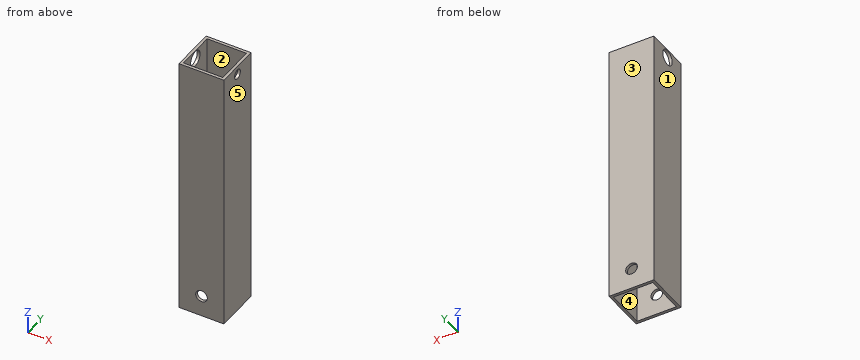
```python
from build123d import *

# Parameters (mm, degrees)
SKETCH1_W                      = 25.4
SKETCH1_H                      = 25.4
BOSS_EXTRUDE1_DEPTH            = 74.93
SHELL1_T                       = -1.5875
CBORE_FOR_M5_SHCS1_D           = 5.5
CBORE_FOR_M5_SHCS1_CBORE_D     = 8.8
CBORE_FOR_M5_SHCS1_CBORE_DEPTH = 5
M6_CLEARANCE_HOLE1_D           = 6.6


with BuildPart() as part:
    # Sketch1 → Boss-Extrude1 (new body, symmetric)
    with BuildSketch(Plane.XY):
        Rectangle(SKETCH1_W, SKETCH1_H)
    extrude(amount=BOSS_EXTRUDE1_DEPTH, both=True)

    # Shell1
    shell1_openings = [part.faces().sort_by_distance(p)[0] for p in [
        (0, 0, 74.93),
        (0, 0, -74.93),
    ]]
    offset(amount=SHELL1_T, openings=shell1_openings, kind=Kind.INTERSECTION)

    # CBORE for M5 SHCS1 (through all)
    with Locations(Plane.ZY.offset(12.7)):
        with Locations((70.1675, 0)):
            CounterBoreHole(CBORE_FOR_M5_SHCS1_D / 2, CBORE_FOR_M5_SHCS1_CBORE_D / 2, CBORE_FOR_M5_SHCS1_CBORE_DEPTH)

    # M6 Clearance Hole1 (through all)
    with Locations(Plane(origin=(0, -12.7, 0), x_dir=(-1, 0, 0), z_dir=(0, -1, 0))):
        with Locations((0, 62.93)):
            Hole(M6_CLEARANCE_HOLE1_D / 2)


solid = part.part
```
Can you work these out from the model? Positions are in its coordinate system, mm. Face numbers are marked on the shaded views. A direction names the side the tool comes from. Coordinates: 2 decimals unless noted, no trailing zeros. Loops run counter-clockwise (first coordinate to the right, second up) from the corner with the lowest first, then second, coordinate; pieces in that order, holes last.
Item 1: If we mould it in two halves opening along X, with no side actions, what happens to the marked faces 3, 4 and 5? For each: released by +X, released by -X, zero draft, split by the parting line, or undercut.
Answers below:
face 3: zero draft
face 4: undercut
face 5: released by +X
Item 2: Please list where these lines run through material, in increasing order: L1, parallel to Y at x = -11, z = -12; L2, parallel to X at y = 11.9, z = -62.93.
Answers below:
L1: y = -12.7 to -11.11, 11.11 to 12.7
L2: x = -12.7 to -3.3, 3.3 to 12.7
Item 3: Suppose I cut it at D-D (z = 64.5). Please give me the cut outline in (x, y), then the cut area to 3 significant figures.
Answers below:
outline: (-12.7, -12.7) - (12.7, -12.7) - (12.7, 12.7) - (-12.7, 12.7) - close; hole (-11.11, -11.11) - (11.11, -11.11) - (11.11, 11.11) - (-11.11, 11.11) - close
area: 151 mm2
Item 4: Suppose I cut it at C-C (y = 0). Please give me the cut outline in (x, z).
Answers below:
outline: (-12.7, -74.93) - (-11.11, -74.93) - (-11.11, 65.77) - (-12.7, 65.77) - close; (-12.7, 74.57) - (-11.11, 74.57) - (-11.11, 74.93) - (-12.7, 74.93) - close; (11.11, -74.93) - (12.7, -74.93) - (12.7, 67.42) - (11.11, 67.42) - close; (11.11, 72.92) - (12.7, 72.92) - (12.7, 74.93) - (11.11, 74.93) - close
Item 5: Suppose I cut it at A-A (x = 0). Please give me the cut outline in (y, z), then the cut area to 3 significant figures.
Answers below:
outline: (-12.7, -74.93) - (-11.11, -74.93) - (-11.11, -66.23) - (-12.7, -66.23) - close; (-12.7, -59.63) - (-11.11, -59.63) - (-11.11, 74.93) - (-12.7, 74.93) - close; (11.11, -74.93) - (12.7, -74.93) - (12.7, -66.23) - (11.11, -66.23) - close; (11.11, -59.63) - (12.7, -59.63) - (12.7, 74.93) - (11.11, 74.93) - close
area: 455 mm2
Item 6: Suppose I cut it at B-B (z = -62.93). Please give me the cut outline in (x, y).
Answers below:
outline: (-12.7, -12.7) - (-3.3, -12.7) - (-3.3, -11.11) - (-11.11, -11.11) - (-11.11, 11.11) - (-3.3, 11.11) - (-3.3, 12.7) - (-12.7, 12.7) - close; (3.3, -12.7) - (12.7, -12.7) - (12.7, 12.7) - (3.3, 12.7) - (3.3, 11.11) - (11.11, 11.11) - (11.11, -11.11) - (3.3, -11.11) - close
Item 7: Which directions (+Z, -Z, +X, -X, +Y, -Y) give clear straight access to the entire face, cutting with the end or side of a thin tool? Please do the marked faces 1 and 2.
Answers below:
face 1: +Z, -Z, -X, +Y, -Y
face 2: +Z, -Z
